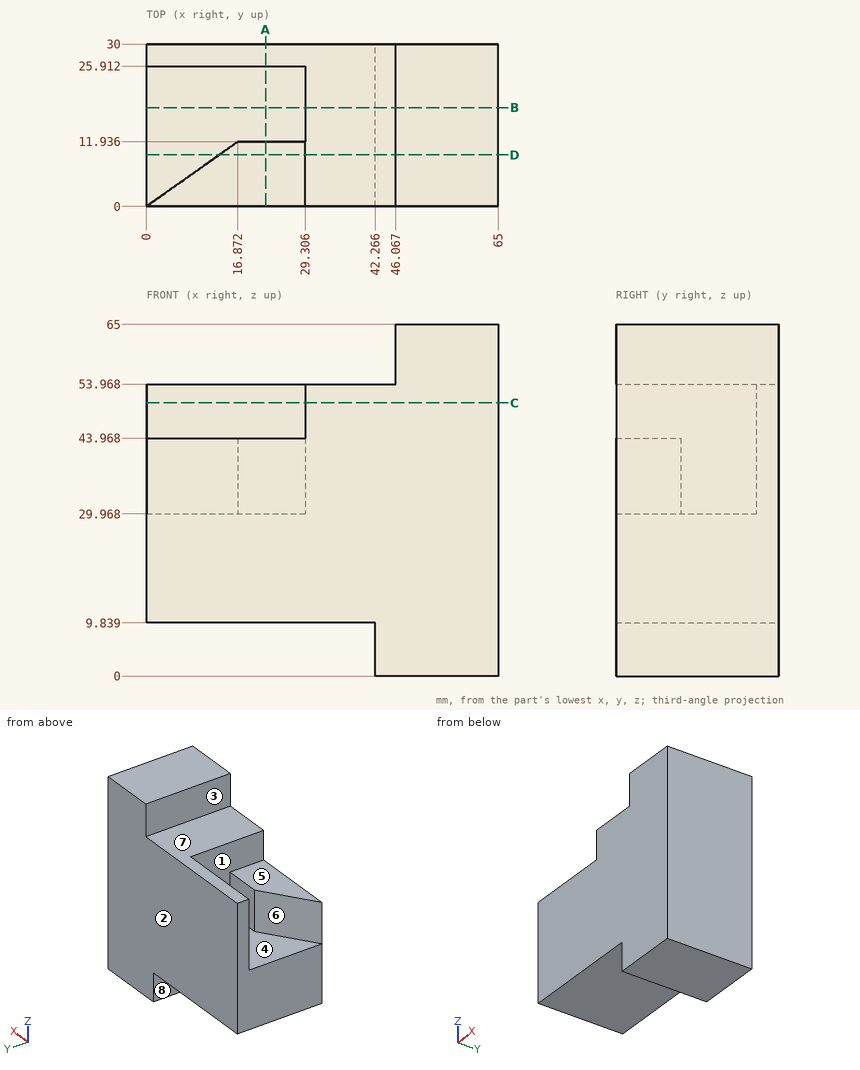
Input: dimensioned drawing with shaded views. Units: mm. Origin: part minimum x, y, z. A direction names the side the tool comes from. Coordinates: 2 decimals unless noted, no trailing zeros. Order: outer loops, then holes, each group sorted by start corner. A loop starts at its lowest first (then second) coordinate and runs counter-clockwise, first axis right, second up.
1. Cut plane C-C, the plane z = 50.5. Return loops of the section in (x, y).
Checked values:
outline: (0, 25.91) - (29.31, 25.91) - (29.31, 0) - (65, 0) - (65, 30) - (0, 30) - close
2. Access query for the marked faces 5, 6, 7 and 8. Directions: +Z, -Z, +X, -X, +Y, -Y. A direction counts if a zero-diameter tool reaches every point of the face in a straight line with its end or side. Return the directions, or none.
Checked values:
face 5: +Z, -X, -Y
face 6: +Z, -X
face 7: +Z, -X, +Y, -Y
face 8: -Z, -X, +Y, -Y
3. Cut plane A-A, the plane x = 22. Return loops of the section in (y, z) (1 decimal), plus the area to 3 significant figures.
Checked values:
outline: (0, 9.8) - (30, 9.8) - (30, 54) - (25.9, 54) - (25.9, 30) - (11.9, 30) - (11.9, 44) - (0, 44) - close
area: 869 mm2
4. Draft query along Y for the marked faces 1, 2, 3 and 4. Return one class per face: +Y half, -Y half, draft (parallel to the pull), parting line (faces both ways), or undercut.
Checked values:
face 1: undercut
face 2: +Y half
face 3: draft
face 4: undercut
5. Contact query for flat-ended pins moving along their axis: P1, Ø9, axis at y = 18.5, z = 58, coming from the -X side; P2, Ø5, axis at x = 32.5, y = 12, coming from the +Z side; P3, Ø7, axis at y = 7, z = 45, coming from the -X side (1 decimal); P4, Ø1, axis at x = 28.5, z = 55.5, coming from the -Y side. Output: stop coordinate, or through.
Checked values:
P1: stops at x = 29.31
P2: stops at z = 53.97
P3: stops at x = 5.2
P4: passes through
6. Ray query, line 1 along Y through (x, z) = (17.5, 41) (1 decimal); line 2 along X through (y, z) = (17.25, 32.5); line 3 along Z through (x, y) = (35.5, 5.5). Return the intervals inside material, ascending.
Checked values:
line 1: y = 0 to 11.9, 25.9 to 30
line 2: x = 29.31 to 65
line 3: z = 9.84 to 53.97
7. Cut plane B-B, the plane y = 18.25. Return loops of the section in (x, z).
Checked values:
outline: (0, 9.84) - (42.27, 9.84) - (42.27, 0) - (65, 0) - (65, 65) - (46.07, 65) - (46.07, 53.97) - (29.31, 53.97) - (29.31, 29.97) - (0, 29.97) - close
8. Cut plane D-D, the plane y = 9.5. Return loops of the section in (x, z).
Checked values:
outline: (0, 9.84) - (42.27, 9.84) - (42.27, 0) - (65, 0) - (65, 65) - (46.07, 65) - (46.07, 53.97) - (29.31, 53.97) - (29.31, 43.97) - (13.43, 43.97) - (13.43, 29.97) - (0, 29.97) - close
